from build123d import *

# Parameters (mm, degrees)
CROQUIS1_W              = 38.1
CROQUIS1_H              = 6.31
SALIENTE_EXTRUIR1_DEPTH = 228.31
CROQUIS2_W              = 38.1
CROQUIS2_H              = 6.31
SALIENTE_EXTRUIR2_DEPTH = 790.55
CROQUIS3_W              = 38.1
CROQUIS3_H              = 6.31
SALIENTE_EXTRUIR3_DEPTH = 324.39
CROQUIS4_R              = 6.35
CORTAR_EXTRUIR1_DEPTH   = 6.31


with BuildPart() as part:
    # Croquis1 → Saliente-Extruir1 (new body)
    with BuildSketch(Plane.XY):
        Rectangle(CROQUIS1_W, CROQUIS1_H)
    extrude(amount=SALIENTE_EXTRUIR1_DEPTH)

    # Croquis2 → Saliente-Extruir2 (add)
    with BuildSketch(Plane(origin=(0, 3.155, 0), x_dir=(1, 0, 0), z_dir=(0, 1, 0))):
        with Locations((0, -225.155)):
            Rectangle(CROQUIS2_W, CROQUIS2_H)
    extrude(amount=SALIENTE_EXTRUIR2_DEPTH)

    # Croquis3 → Saliente-Extruir3 (add)
    with BuildSketch(Plane(origin=(0, 0, 222), x_dir=(-1, 0, 0), z_dir=(0, 0, -1))):
        with Locations((0, 790.55)):
            Rectangle(CROQUIS3_W, CROQUIS3_H)
    extrude(amount=SALIENTE_EXTRUIR3_DEPTH)

    # Croquis4 → Cortar-Extruir1 (cut)
    with BuildSketch(Plane(origin=(0, 793.705, 0), x_dir=(1, 0, 0), z_dir=(0, 1, 0))):
        with Locations(Location((0, 90.497795334, 0), (0, 0, 180))):
            Circle(CROQUIS4_R)
        with Locations(Location((0, 58.497795334, 0), (0, 0, 180))):
            Circle(CROQUIS4_R)
    extrude(amount=-CORTAR_EXTRUIR1_DEPTH, mode=Mode.SUBTRACT)


solid = part.part
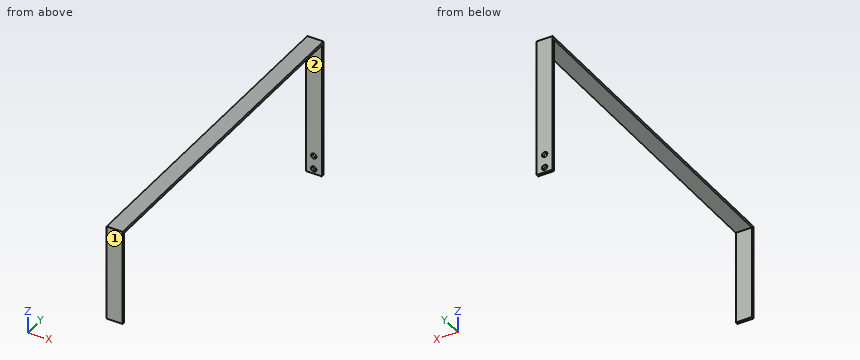
Read the model definition and answer for the solid it produces. Units are mm, in the model's axes. Face numbers are marked on the shaded views. A direction names the side the tool comes from. Give positions to 0.01 mm unless a question says otherwise; leave off trailing zeros. Write each loop counter-clockwise with the first axis right and the second up, starting at its lowest first coordinate (ties: lowest second). Pieces come first, ordered by that corner, then holes. Notation, with made-up numbers: (10.25, 15) - (33.25, 15) arc R28 cw to (33.25, 37) - close; hole circle Ø1 at (2, -10). An arc over 180 degrees is marked (long way). Return JSON: item names as keys, results as strings.
Q1. A cutting plane is placed at C-C, the plane y = 668.5. Determine the outline of the cut face in (x, z), and give its area (3 significant figures).
Reply:
{"outline": "(-19.05, 222) - (19.05, 222) - (19.05, 228.31) - (-19.05, 228.31) - close", "area": "240 mm²"}
Q2. Given P1, Ø5, axis at x = 2.5, y = 597.5, coming from the -Z side; P2, Ø7, axis at x = -3.5, y = 0, coming from the -Z side, each flat-ended and moving along its own axis, determine where each tip first touches the part or whether it passes through.
Reply:
{"P1": "z = 222", "P2": "z = 0"}
Q3. Consider line 1 along Z through (x, y) = (0, 790); line 2 along Y through (x, z) = (15, 198.5) (3 decimals); line 3 along Y through (x, z) = (-0.5, -35) (3 decimals). Determine where each line is inside the solid, lowest interval first. Write a range as [from, to].
Reply:
{"line 1": "[-102.39, -96.85], [-84.15, -64.85], [-52.15, 228.31]", "line 2": "[-3.155, 3.155], [787.395, 793.705]", "line 3": "[787.395, 793.705]"}
Q4. For the marked faces 1 and 2, determine the directions among +Z, -Z, +X, -X, +Y, -Y from which every point of the face is accessible in a straight line to the end or side of a thin tool.
Reply:
{"face 1": "+Z, -Z, +X, -X, -Y", "face 2": "-Z, +X, -X"}
Q5. A cutting plane is placed at B-B, the plane z = 161. Determine the outline of the cut face in (x, y) (3 decimals).
Reply:
{"outline": "(-19.05, -3.155) - (19.05, -3.155) - (19.05, 3.155) - (-19.05, 3.155) - close; (-19.05, 787.395) - (19.05, 787.395) - (19.05, 793.705) - (-19.05, 793.705) - close"}
Q6. A cutting plane is placed at A-A, the plane x = 0. Determine the outline of the cut face in (y, z) (3 decimals).
Reply:
{"outline": "(-3.155, 0) - (3.155, 0) - (3.155, 222) - (787.395, 222) - (787.395, -52.148) - (793.705, -52.148) - (793.705, 228.31) - (-3.155, 228.31) - close; (787.395, -102.39) - (793.705, -102.39) - (793.705, -96.848) - (787.395, -96.848) - close; (787.395, -84.148) - (793.705, -84.148) - (793.705, -64.848) - (787.395, -64.848) - close"}
